Check sheet for the modelled part. Datum: model origin and axes. Units: mm. Face numbers are marked on the shaded views. A direction names the side the tool comes from. Give positions to 0.01 mm unless a question says otherwise; leave off trailing zeros. Write each loop counter-clockwise with the first axis right and the second up, starting at its lowest first coordinate (ties: lowest second). Pieces come first, ordered by that corner, then holes. Notation, with made-up numbers: (89, -5.75) -> (114, -5.75) arc R10 cw to (114, 7.25) -> close; hole circle Ø7 at (-5.75, -21). An arc over 180 degrees is marked (long way). Answer as a JSON object with one key per item and string values.
from build123d import *

# Parameters (mm, degrees)
BOSS_EXTRUDE1_DEPTH = 4.7625
SKETCH2_R           = 6.35
BOSS_EXTRUDE2_DEPTH = 9.525
FILLET1_R           = 2.54
FILLET2_START       = -4.7625
FILLET2_DEPTH       = 9.525


with BuildPart() as part:
    # Sketch1 → Boss-Extrude1 (new, symmetric)
    with BuildSketch(Plane.XY):
        with BuildLine():
            ThreePointArc((22.094337813, 8.067740847), (24.226136754, 10.836108919), (26.914852205, 13.067529481))
            Line((26.914852205, 13.067529481), (32.554450869, 13.067529481))
            Line((32.554450869, 13.067529481), (17.117145822, -12.379943283))
            Line((17.117145822, -12.379943283), (17.117145822, -24.9994))
            Line((17.117145822, -24.9994), (11.719856102, -24.9994))
            ThreePointArc((11.719856102, -24.9994), (9.533586303, -22.160148794), (10.767145822, -18.795709173))
            Line((10.767145822, -18.795709173), (10.767145822, -10.604456717))
            Line((10.767145822, -10.604456717), (22.094337813, 8.067740847))
        make_face()
    extrude(amount=BOSS_EXTRUDE1_DEPTH, both=True)

    # Sketch2 → Boss-Extrude2 (add, through all)
    with BuildSketch(Plane.XY.offset(4.7625)):
        with Locations((13.942145822, -11.4922)):
            Circle(SKETCH2_R)
    extrude(amount=-BOSS_EXTRUDE2_DEPTH)

    # Sketch3 → 9/64 (0.14063) Diameter Hole1 (revolve, cut)
    with BuildSketch(Plane(origin=(13.942145822, -11.4922, 4.7625), x_dir=(0, -1, 0), z_dir=(1, 0, 0))):
        Polygon((0, 0), (0, 9.525), (2.421001, 9.525), (1.786001, 8.89), (1.786001, 0.635), (2.421001, 0), align=None)
    revolve(axis=Axis((13.942145822, -11.4922, 11.1125), (0, 0, -1)), mode=Mode.SUBTRACT)

    # Fillet1
    fillet1_edges = [part.edges().sort_by_distance(p)[0] for p in [
        (26.914852205, 13.067529481, 0),
        (32.554450869, 13.067529481, 0),
        (17.117145822, -24.9994, 0),
        (11.719856102, -24.9994, 0),
        (14.079831445, -5.143692879, 0),
        (17.117145822, -16.991461314, 0),
        (19.508957077, -8.437185686, 0),
    ]]
    fillet(fillet1_edges, radius=FILLET1_R)

    # Fillet2: read off the stored shape, not the designer's step
    # Fillet2 outline → Fillet2 (add)
    with BuildSketch(Plane.XY.offset(FILLET2_START)):
        with BuildLine():
            add(Edge.make_bspline(
                [(10.767145822, -18.017877519), (10.767145823, -17.393004157), (10.487472268, -16.852808402), (10.023052756, -16.488519599)],
                knots=[0.43435667, 0.43435667, 0.43435667, 0.43435667, 1, 1, 1, 1], degree=3, weights=[0.852569416, 0.837715519, 0.886859046, 1]))
            Line((10.767145822, -18.017877519), (10.767145822, -16.991461314))
            ThreePointArc((10.767145822, -16.991461314), (10.386196343, -16.753162203), (10.023052756, -16.488519599))
        make_face()
        with BuildLine():
            add(Edge.make_bspline(
                [(10.328377861, -19.24798429), (10.606973983, -18.907141934), (10.767145822, -18.483132326), (10.767145822, -18.017877519)],
                knots=[0, 0, 0, 0, 0.43435667, 0.43435667, 0.43435667, 0.43435667], degree=3, weights=[1, 0.91311923, 0.863975702, 0.852569416]))
            ThreePointArc((10.328377861, -19.24798429), (10.538145849, -19.01251792), (10.767145822, -18.795709173))
            Line((10.767145822, -18.795709173), (10.767145822, -18.017877519))
        make_face()
    extrude(amount=FILLET2_DEPTH)


solid = part.part
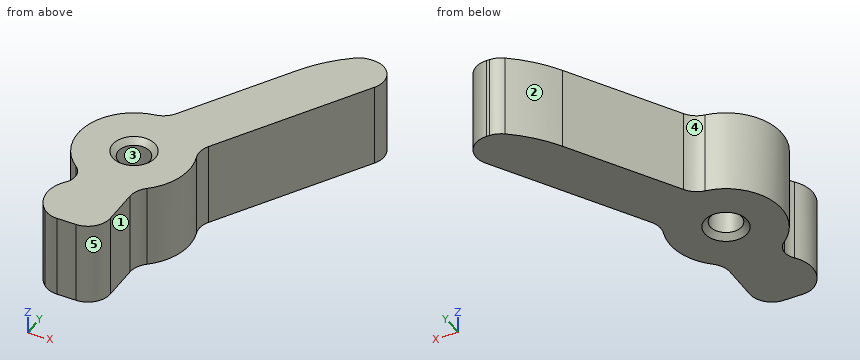
1. Sectioned sample at B-B, the plane x = 23.5. Enter the section's corners in (y, z).
Determined:
{"outline": "(-1.86, -4.76) -> (10.03, -4.76) -> (10.03, 4.76) -> (-1.86, 4.76) -> close"}
2. Sectioned sample at A-A, the plane y = -4.5. Enter the section's corners in (x, z).
Determined:
{"outline": "(14.39, -4.76) -> (21.9, -4.76) -> (21.9, 4.76) -> (14.39, 4.76) -> close"}
3. Access from +Z, -Z, +X, -X, +Y, -Y to the whole of each face (thin tool, end or side, straight path). Record for the marked faces 1 and 2.
Determined:
{"face 1": "+Z, -Z, +X, -Y", "face 2": "+Z, -Z, -X, +Y"}
4. Scan lines: L1, parallel to X at y = -11.5, z = -2.25; L2, parallel to Y at x = 23, z = 1.5; L3, parallel to Y at x = 11.5, z = -0.5. Record each from-to range of solid material in increasing order. Write a range as [from, to].
Determined:
{"L1": "[7.59, 12.16], [15.73, 20.29]", "L2": "[-2.68, 9.4]", "L3": "[-24.83, -5.63]"}
5. Go/stop test with flat-tipped pins: P1, Ø3, axis at x = 11, z = 0.5, coming from the +Y side; P2, Ø4.5, axis at y = -20.5, z = 0.5, coming from the +X side; P3, Ø2, axis at y = -20.5, z = 2.5, coming from the -X side; P4, Ø3, axis at x = 13.94, y = -11.49, coming from the -Z side. Record where each tip stops, or that it passes through.
Determined:
{"P1": "y = -5.31", "P2": "x = 17.12", "P3": "x = 9.49", "P4": "through"}
6. Mould release check, pull along X, two halves, no side actions. Record for the marked faces 3, 4 and 5: released by +X, released by -X, zero draft, split by the parting line, or undercut.
Determined:
{"face 3": "undercut", "face 4": "released by -X", "face 5": "released by +X"}
